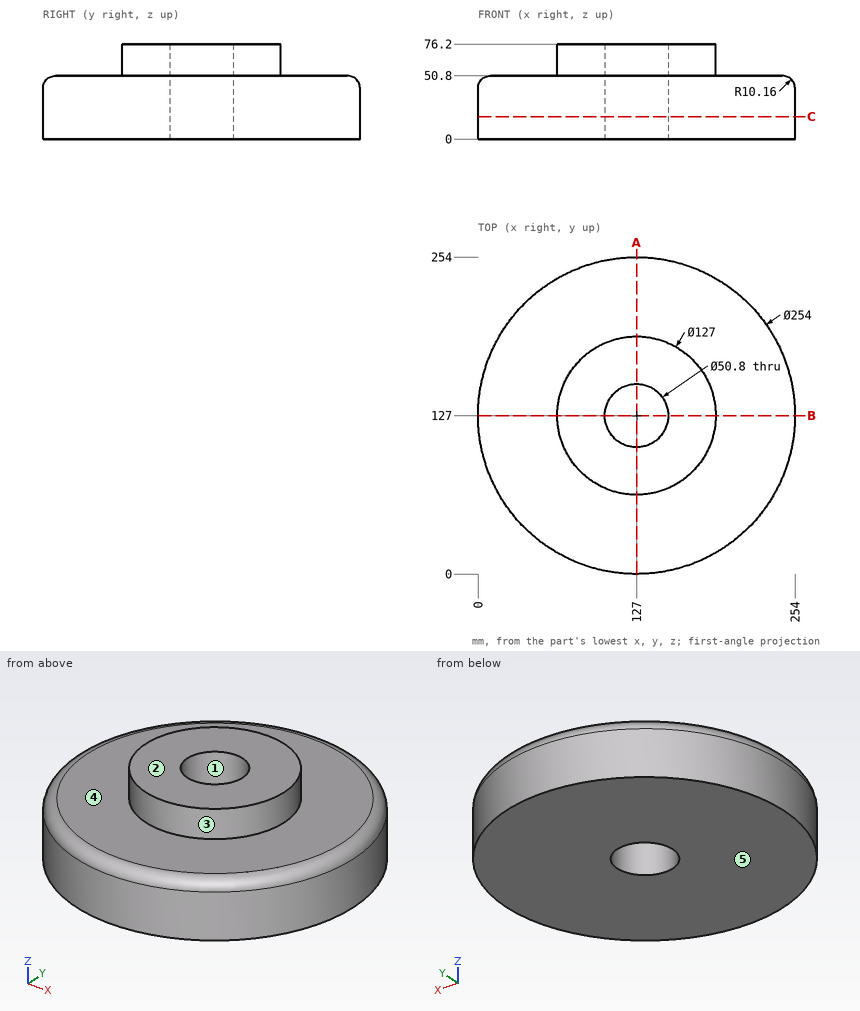
Part print with two shaded views. Sizes in mm from the minimum x, y, z corner. A direction names the side the tool comes from. Coordinates: 2 decimals unless noted, no trailing zeros. Order: outer loops, then holes, each group sorted by start corner. A loop starts at its lowest first (then second) coordinate and runs counter-clockwise, first axis right, second up.
(1) Mould opens along X. For the marked faces 1, 2 and 3 say: released by +X, released by -X, zero draft, split by the parting line, or undercut.
Solution:
face 1: undercut
face 2: zero draft
face 3: split by the parting line
(2) Saw through at A-A, the plane x = 127. Write the cut outline in (y, z), and give its area (3 significant figures).
Solution:
outline: (0, 0) - (101.6, 0) - (101.6, 76.2) - (63.5, 76.2) - (63.5, 50.8) - (10.16, 50.8) arc R10.16 ccw to (0, 40.64) - close; (152.4, 0) - (254, 0) - (254, 40.64) arc R10.16 ccw to (243.84, 50.8) - (190.5, 50.8) - (190.5, 76.2) - (152.4, 76.2) - close
area: 12,200 mm2
(3) Saw through at C-C, the plane z = 18. Write the cut outline in (x, y), and give its area (3 significant figures).
Solution:
outline: circle Ø254 at (127, 127); hole circle Ø50.8 at (127, 127)
area: 48,600 mm2
(4) Which spindle directions (+Z, -Z, +X, -X, +Y, -Y) get a long thin tool onto all of the face, cutting with end or side? Do the marked faces 4 and 5. Say none if no direction does.
Solution:
face 4: +Z
face 5: -Z, +X, -X, +Y, -Y
(5) Drill centre lines: L1, parallel to Y at x = 127, z = 61.5; L2, parallel to Y at x = 127, z = 37; L3, parallel to Z at x = 197.5, y = 134.5. Where is each one in solid material? Low to high.
Solution:
L1: y = 63.5 to 101.6, 152.4 to 190.5
L2: y = 0 to 101.6, 152.4 to 254
L3: z = 0 to 50.8
(6) Pin check, flat tips, straight feed: pin 1 Ø8 at (y, z) = (183, 51.5) entering from +X; pin 2 Ø12 at (x, y) = (100, 26) entering from +Z; pin 3 Ø10 at (x, z) = (183, 8.5) entering from +Y. Stop position of each tip, or through.
Solution:
pin 1: stops at x = 238.45
pin 2: stops at z = 50.8
pin 3: stops at y = 243.31
